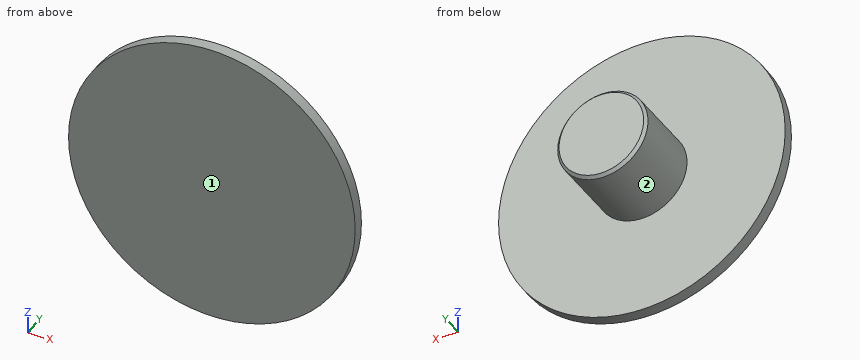
Autodesk Fusion 360 part; units mm, degrees
sketch "Sketch1" plane through (0, 0, 0) normal (0, 1, 0) x (1, 0, 0)
  circle A0 centre (0, 0) radius 12.7
  circle A1 centre (0, 0) radius 4
  dimension "d1" = 25.4
  dimension "d4" = 8
extrude "Extrude1" add sketch "Sketch1" along normal blind 1
extrude "Extrude2" add sketch "Sketch1" along normal blind 7.5 contours A1
chamfer "Chamfer1" distance 0.25 angle 45 1 edges at (-3.7293, 7.5, 1.4465)
equation "d5 = 10.5 mm - 3 mm"
Can you work these out from the model? Positions are in its coordinate system, mm. Face numbers are marked on the shaded views. A direction names the side the tool comes from. Give positions to 0.01 mm unless a question says otherwise; leave off trailing zeros. Order: outer loops, then holes, each group sorted by start corner. A loop starts at its lowest first (then second) coordinate and runs counter-clockwise, first axis right, second up. Notation, with made-up numbers: M 44.25,-1.75 L 79.25,-1.75 A24 cw 79.25,25.25 Z; hole C -28.75,22 d7. An arc over 180 degrees is marked long. Use a Markdown table: item, result. Add a question column.
Item 1: Suppose I cut it at C-C (y = 4). List the corners of the cut face in (x, z) for me.
Item 2: Suppose I cut it at B-B (x = 0). List the corners of the cut face in (y, z) for me, then the cut area to 3 significant figures.
Item 3: Will these pins go through, and if not, where does the flat tip stop? pin 1 (5 mm diameter, centred on x = 8.5, z = 4.5, fed in from +Y); pin 2 (3 mm diameter, centred on y = 2, z = 5.5, fed in from -X); pin 3 (2 mm diameter, centred on x = -4.5, y = 4.5, fed in from +Z).
Item 4: For the marked faces 1 and 2, which set-ups out of +Z, -Z, +X, -X, +Y, -Y let a thin tool reach every point of the face, with its end or its side?
Item 5: Suppose I cut it at D-D (z = 7.25). List the corners of the cut face in (x, y) for me.
Item 6: Suppose I cut it at A-A (z = 0). List the corners of the cut face in (x, y) for me.
Item 7: If I drill on L1, parallel to Y at x = 3.25, z = 5.5; L2, parallel to X at y = 4, z = -0.25; L3, parallel to Y at x = 3, z = -2.5, over which ranges is the centre line in solid material (lowest first)? Write a range as [from, to].
Answer sheet:
| question | item | result |
|---|---|---|
| 1 | outline | C 0,0 d8 |
| 2 | outline | M 0,-12.7 L 1,-12.7 L 1,-4 L 7.25,-4 L 7.5,-3.75 L 7.5,3.75 L 7.25,4 L 1,4 L 1,12.7 L 0,12.7 Z |
| 2 | area | 77.3 mm² |
| 3 | pin 1 | stops at y = 1 |
| 3 | pin 2 | stops at x = -11.92 |
| 3 | pin 3 | stops at z = 1.94 |
| 4 | face 1 | +Z, -Z, +X, -X, -Y |
| 4 | face 2 | +Y |
| 5 | outline | M -10.43,0 L 10.43,0 L 10.43,1 L -10.43,1 Z |
| 6 | outline | M -12.7,0 L 12.7,0 L 12.7,1 L 4,1 L 4,7.25 L 3.75,7.5 L -3.75,7.5 L -4,7.25 L -4,1 L -12.7,1 Z |
| 7 | L1 | y = [0, 1] |
| 7 | L2 | x = [-3.99, 3.99] |
| 7 | L3 | y = [0, 7.34] |
